Build history of the part. All positions in model axes, mm. A direction names the side the tool comes from. Give positions to 0.01 mm unless a question says otherwise; leave off trailing zeros. Order: outer loops, then holes, each group sorted by start corner. A loop starts at its lowest first (then second) coordinate and runs counter-clockwise, first axis right, second up. Notation, with made-up numbers: M 51.5,-23.5 L 62.5,-23.5 A32 cw 62.5,13.5 Z; hole C -28,-36 d10. An arc over 180 degrees is marked long. Answer as CSV lines item,"result".
from build123d import *

# Parameters (mm, degrees)
SKETCH1_W                               = 250
SKETCH1_H                               = 90
BOSS_EXTRUDE1_DEPTH                     = 20
CUT_EXTRUDE1_DEPTH                      = 158.876534038
CUT_EXTRUDE1_DEPTH_BACK                 = 158.876534038
SKETCH11_R                              = 29
CBORE_FOR_M5_HEX_HEAD_BOLT2_D           = 5.5
CBORE_FOR_M5_HEX_HEAD_BOLT2_CBORE_D     = 10.5
CBORE_FOR_M5_HEX_HEAD_BOLT2_CBORE_DEPTH = 6
SKETCH15_R                              = 32.75
CUT_EXTRUDE2_DEPTH                      = 13


with BuildPart() as part:
    # Sketch1 → Boss-Extrude1 (new body)
    with BuildSketch(Plane(origin=(0, 0, 0), x_dir=(1, 0, 0), z_dir=(0, 1, 0))):
        with Locations((25, 0)):
            Rectangle(SKETCH1_W, SKETCH1_H)
    extrude(amount=BOSS_EXTRUDE1_DEPTH)

    # Sketch11 → Cut-Extrude1 (cut, two sides: drawn at the far end of the back side and taken through both)
    with BuildSketch(Plane(origin=(0, 20, 0), x_dir=(1, 0, 0), z_dir=(0, 1, 0)).offset(-CUT_EXTRUDE1_DEPTH_BACK)):
        with Locations(Location((0, 0, 0), (0, 0, 270))):
            Circle(SKETCH11_R)
    extrude(amount=CUT_EXTRUDE1_DEPTH + CUT_EXTRUDE1_DEPTH_BACK, mode=Mode.SUBTRACT)

    # CBORE for M5 Hex Head Bolt2 (through all)
    with Locations(Plane(origin=(-32.335783638, 20, -13.393920133), x_dir=(0, 0, 1), z_dir=(0, 1, 0))):
        with Locations((0, 0), (-18.941863505, 18.941863505), (-18.941863505, 45.729703771), (0, 64.671567276), (26.787840266, 64.671567276), (45.729703771, 45.729703771), (45.729703771, 18.941863505), (26.787840266, 0)):
            CounterBoreHole(CBORE_FOR_M5_HEX_HEAD_BOLT2_D / 2, CBORE_FOR_M5_HEX_HEAD_BOLT2_CBORE_D / 2, CBORE_FOR_M5_HEX_HEAD_BOLT2_CBORE_DEPTH)

    # Sketch15 → Cut-Extrude2 (cut)
    with BuildSketch(Plane(origin=(0, 0, 0), x_dir=(1, 0, 0), z_dir=(0, 1, 0))):
        Circle(SKETCH15_R)
    extrude(amount=CUT_EXTRUDE2_DEPTH, mode=Mode.SUBTRACT)


solid = part.part
Item 1: Probe line 1 along X through (y, z) = (6.25, 1.5); line 2 along X through (y, z) = (6, -29.5); line 3 along Z through (x, y) = (-33.5, 8.5). List the from-to ranges inside material, lowest first. Write a range as from..to.
Geometry says:
line 1,"x = -100..-32.72, 32.72..150"
line 2,"x = -100..-14.22, 14.22..150"
line 3,"z = -45..-15.89, -10.9..10.9, 15.89..45"
Item 2: Band-saw the part on A-A (x = 0). Give the cut face in (y, z), and give its area (4 significant figures).
Geometry says:
outline,"M 0,-45 L 20,-45 L 20,-29 L 13,-29 L 13,-32.75 L 0,-32.75 Z; M 0,32.75 L 13,32.75 L 13,29 L 20,29 L 20,45 L 0,45 Z"
area,"542.5 mm2"
Item 3: Pull direction Z, two halves, no side cores. Call faces 1 (the flat face through (23, 10, -45)), 2 (the flat face through (23, 10, 45)), 3 (the flat face through (-35, 14, -11)): released by +Z, released by -Z, zero draft, split by the parting line, or undercut.
Geometry says:
face 1,"released by -Z"
face 2,"released by +Z"
face 3,"undercut"
Item 4: Drop flat-ended pins along their axis: pin 1 (6.5 mm diameter, centred on x = 32.34, z = -13.39, fed in from +Y); pin 2 (4.5 mm diameter, centred on x = -13.39, z = -32.34, fed in from +Y). Give the stop position or say it passes through.
Geometry says:
pin 1,"stops at y = 14"
pin 2,"passes through"
Item 5: Band-saw the part on C-C (y = 2.25). Give the cut face in (x, z).
Geometry says:
outline,"M -100,-45 L 150,-45 L 150,45 L -100,45 Z; hole M -30.81,-11.11 A2.75 ccw long -29.64,-13.93 A32.75 ccw -13.93,-29.64 A2.75 ccw long -11.11,-30.81 A32.75 ccw 11.11,-30.81 A2.75 ccw long 13.93,-29.64 A32.75 ccw 29.64,-13.93 A2.75 ccw long 30.81,-11.11 A32.75 ccw 30.81,11.11 A2.75 ccw long 29.64,13.93 A32.75 ccw 13.93,29.64 A2.75 ccw long 11.11,30.81 A32.75 ccw -11.11,30.81 A2.75 ccw long -13.93,29.64 A32.75 ccw -29.64,13.93 A2.75 ccw long -30.81,11.11 A32.75 ccw Z"
Item 6: 3-axis set-ups, long thin cutter, end or side, ignore diameter. For faces 4 (the cylindrical face through (-23.27, 6.409, 23.045)), 5 (the flat face through (-16, 14, -30)), 6 (the flat face through (150, 10, 1)): which of +Z, -Z, +X, -X, +Y, -Y reach the whole face in a straight line?
Geometry says:
face 4,"-Y"
face 5,"+Y"
face 6,"+Z, -Z, +X, +Y, -Y"
Item 7: Band-saw the part on B-B (z = 0). Give the cut face in (x, y), and give its area (3 significant figures).
Geometry says:
outline,"M -100,0 L -32.75,0 L -32.75,13 L -29,13 L -29,20 L -100,20 Z; M 29,13 L 32.75,13 L 32.75,0 L 150,0 L 150,20 L 29,20 Z"
area,"3,740 mm2"
